Autodesk Inventor part; units mm, degrees
ref_plane "Work Plane1" through (3.175, 0, 0) normal (1, 0, 0) x (0, 1, 0)
ref_plane "XZ Plane" through (0, 0, 0) normal (0, 1, 0) x (-1, 0, 0)
ref_plane "XY Plane" through (0, 0, 0) normal (0, 0, 1) x (1, 0, 0)
ref_plane "Work Plane1" through (3.175, 0, 0) normal (1, 0, 0) x (0, 1, 0)
sketch "Sketch1" plane through (3.175, 0, 0) normal (1, 0, 0) x (0, 1, 0)
  line L0 (93.6959, 280.1689) -> (17.4959, 280.1689)
  line L1 (17.4959, 280.1689) -> (17.4959, 153.1689)
  line L2 (17.4959, 153.1689) -> (93.6959, 153.1689)
  line L3 (93.6959, 153.1689) -> (93.6959, 280.1689)
  point P0 (0, 0)
  dimension "d1" = 127
  dimension "d2" = 76.2
extrude "Extrusion1" add sketch "Sketch1" along normal blind 25.4
sketch "Sketch2" plane through (28.575, 0, 0) normal (1, 0, 0) x (0, 0, -1)
  circle A0 centre (-270.0089, 27.6559) radius 6.35
  line L0 (-280.1689, 93.6959) -> (-280.1689, 17.4959)
  line L1 (-280.1689, 17.4959) -> (-153.1689, 17.4959)
  line L2 (-153.1689, 17.4959) -> (-153.1689, 93.6959)
  line L3 (-153.1689, 93.6959) -> (-280.1689, 93.6959)
  circle A1 centre (-165.8689, 83.5359) radius 6.35
  circle A2 centre (-165.8689, 83.5359) radius 6.35
  circle A3 centre (-165.8689, 83.5359) radius 6.35
  line L4 (-153.1689, 17.4959) -> (-153.1689, 93.6959)
  circle A4 centre (-267.4689, 80.9959) radius 6.35
  circle A5 centre (-163.3289, 27.6559) radius 6.35
  point P0 (0, 0)
  dimension "d5" = 12.7
  dimension "d6" = 10.16
  dimension "d7" = 10.16
  dimension "d8" = 10.16
  dimension "d9" = 12.7
  dimension "d10" = 12.7
  dimension "d11" = 12.7
  dimension "d12" = 12.7
  dimension "d13" = 12.7
  dimension "d14" = 12.7
  dimension "d15" = 10.16
  dimension "d16" = 10.16
extrude "Extrusion2" add sketch "Sketch2" along normal blind 76.2 contours A0 | A1 | A4 | A5
equation "\"d7\" = d6"
equation "\"d8\" = d7"
equation "\"d9\" = d5"
equation "\"d10\" = d5"
equation "\"d11\" = d5"
equation "\"d12\" = d9"
equation "\"d13\" = d12"
equation "\"d14\" = d5"
equation "\"d15\" = d6"
equation "\"d16\" = d6"
properties part number "Table"
CAD build for the part. Positions are in the model's coordinates, mm. A direction names the side the tool comes from. Round coordinates to 2 decimals unless told otherwise and drop trailing zeros. Loops run counter-clockwise (first coordinate to the right, second up) from the corner with the lowest first, then second, coordinate; pieces in that order, holes last. Notation, with made-up numbers: M 56.5,10.5 L 83.5,10.5 A20 cw 83.5,28.5 Z; hole C 19.25,68.5 d5. An arc over 180 degrees is marked long. Use a Markdown table: item, result. Add a question column.
(1) Which spindle directions (+Z, -Z, +X, -X, +Y, -Y) get a long thin tool onto all of the face, cutting with end or side? Do faces 1 (the face through (66.14, 84.86, 272.51)), 2 (the face through (104.775, 28, 270)). Say none if no direction does.
(2) Cut at D-D (z = 271.5). Give the cut face in (x, y) (1 decimal), and give its area (3 significant figures).
(3) Cut at C-C (z = 194). Give the cut face in (x, y) (3 decimals).
(4) Flat gauge pins, fed straight in: pin 1 (1 mm diameter, centred on x = 71.5, z = 265, fed in from +Y); pin 2 (10 mm diameter, centred on y = 56, z = 224.5, fed in from +X) (3 decimals); pin 3 (2 mm diameter, centred on x = 35.5, y = 85, fed in from -Z). Where does each tip first touch, or does it go through?
(5) Pull direction Y, two halves, no side cores. Call faces 3 (the face through (66.142, 30.088, 264.143)), 4 (the face through (16, 93.696, 216)), 5 (the face through (16, 55, 153.169)): +Y half, -Y half, draft (parallel to the pull), parting line (faces both ways), or undercut.
(6) Drill centre lines: line 1 (X direction, y = 45.5, z = 210.5) (3 decimals); line 2 (Z direction, x = 96.5, y = 31.5); line 3 (Y direction, x = 45, z = 267.5). Where is each one in solid material? Low to high.
(7) Cut at A-A (x = 63.5). Give the cut face in (y, z), and give its area (3 significant figures).
(8) Cut at B-B (y = 30). Give the cut face in (x, z) (3 decimals).
Geometry says:
| question | item | result |
|---|---|---|
| 1 | face 1 | +X |
| 1 | face 2 | +Z, -Z, +X, +Y, -Y |
| 2 | outline | M 3.2,17.5 L 28.6,17.5 L 28.6,21.5 L 104.8,21.5 L 104.8,33.8 L 28.6,33.8 L 28.6,76.1 L 104.8,76.1 L 104.8,85.9 L 28.6,85.9 L 28.6,93.7 L 3.2,93.7 Z |
| 2 | area | 3,620 mm² |
| 3 | outline | M 3.175,17.496 L 28.575,17.496 L 28.575,93.696 L 3.175,93.696 Z |
| 4 | pin 1 | stops at y = 87.03 |
| 4 | pin 2 | stops at x = 28.575 |
| 4 | pin 3 | stops at z = 159.54 |
| 5 | face 3 | undercut |
| 5 | face 4 | +Y half |
| 5 | face 5 | draft |
| 6 | line 1 | x = 3.175 to 28.575 |
| 6 | line 2 | z = 158.27 to 168.38, 264.95 to 275.06 |
| 6 | line 3 | y = 21.82 to 33.49, 74.65 to 87.35 |
| 7 | outline | C 27.66,163.33 d12.7; C 27.66,270.01 d12.7; C 81,267.47 d12.7; C 83.54,165.87 d12.7 |
| 7 | area | 507 mm² |
| 8 | outline | M 3.175,153.169 L 28.575,153.169 L 28.575,157.427 L 104.775,157.427 L 104.775,169.23 L 28.575,169.23 L 28.575,264.107 L 104.775,264.107 L 104.775,275.91 L 28.575,275.91 L 28.575,280.169 L 3.175,280.169 Z |
